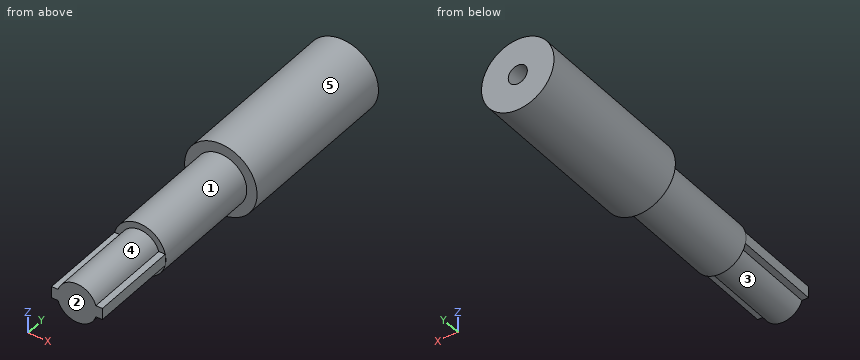
```python
from build123d import *

# Parameters (mm, degrees)
SKETCH1_R           = 3.1
SKETCH1_W           = 8
SKETCH1_H           = 1.8
BOSS_EXTRUDE1_DEPTH = 14
SKETCH2_R           = 4.075
BOSS_EXTRUDE2_DEPTH = 18
SKETCH3_R           = 5.7
BOSS_EXTRUDE3_DEPTH = 2
SKETCH4_R           = 5.7
BOSS_EXTRUDE4_DEPTH = 25
SKETCH5_R           = 1.5
CUT_EXTRUDE1_DEPTH  = 17


with BuildPart() as part:
    # Sketch1 → Boss-Extrude1 (new body)
    with BuildSketch(Plane(origin=(0, 0, 0), x_dir=(1, 0, 0), z_dir=(0, 1, 0))):
        Circle(SKETCH1_R)
        Rectangle(SKETCH1_W, SKETCH1_H)
    extrude(amount=BOSS_EXTRUDE1_DEPTH)

    # Sketch2 → Boss-Extrude2 (add)
    with BuildSketch(Plane(origin=(0, 14, 0), x_dir=(1, 0, 0), z_dir=(0, 1, 0))):
        with Locations(Location((0, 0, 0), (0, 0, 12.759485069))):
            Circle(SKETCH2_R)
    extrude(amount=BOSS_EXTRUDE2_DEPTH)

    # Sketch3 → Boss-Extrude3 (add)
    with BuildSketch(Plane(origin=(0, 32, 0), x_dir=(1, 0, 0), z_dir=(0, 1, 0))):
        with Locations(Location((0, 0, 0), (0, 0, 270))):
            Circle(SKETCH3_R)
    extrude(amount=BOSS_EXTRUDE3_DEPTH)

    # Sketch4 → Boss-Extrude4 (add)
    with BuildSketch(Plane(origin=(0, 34, 0), x_dir=(1, 0, 0), z_dir=(0, 1, 0))):
        with Locations(Location((0, 0, 0), (0, 0, 270))):
            Circle(SKETCH4_R)
    extrude(amount=BOSS_EXTRUDE4_DEPTH)

    # Sketch5 → Cut-Extrude1 (cut)
    with BuildSketch(Plane(origin=(0, 59, 0), x_dir=(1, 0, 0), z_dir=(0, 1, 0))):
        with Locations(Location((0, 0, 0), (0, 0, 270))):
            Circle(SKETCH5_R)
    extrude(amount=-CUT_EXTRUDE1_DEPTH, mode=Mode.SUBTRACT)


solid = part.part
```
The model under review builds one solid part; all positions refer to its coordinate system, in mm. Face numbers are marked on the shaded views. A direction names the side the tool comes from. Give positions to 0.01 mm unless a question says otherwise; leave off trailing zeros. Order: outer loops, then holes, each group sorted by start corner. A loop starts at its lowest first (then second) coordinate and runs counter-clockwise, first axis right, second up. Notation, with made-up numbers: (62, 86.25) - (101, 86.25) arc R12 ccw to (101, 95.25) - close; hole circle Ø5 at (-37.75, 75.25). An arc over 180 degrees is marked (long way). Use CSV: the item, a comma, the result in double quotes. Start each with the question number.
Q1. We need section D-D, the plane y = 33.5. Write out the cut boundary in (x, z), and give its area (3 significant figures).
Q2. Tool access review of the marked faces 4 and 5: name each direction out of +Z, -Z, +X, -X, +Y, -Y from which nothing blocks a thin tool from reaching the whole face with its end or side.
Q3. We need section C-C, the plane y = 45. Write out the cut boundary in (x, z).
Q4. The part is to be moulded in two halves that separate along Z. For the marked faces 1, 2 and 3, say which applies: +Z half, -Z half, draft (parallel to the pull), parting line (faces both ways), or undercut.
Q5. We need section B-B, the plane z = 0. Write out the cut boundary in (x, y) (3 decimals).
Q6. To check wall thickness, follow line 1 along X through (y, z) = (54.5, 0); line 2 along Y through (x, z) = (-3.75, 4.25); line 3 along Z through (x, y) = (0.5, 53.5). State the ranges of each line that lie inside material, in increasing order. Write a range as [from, to].
Q7. Clearance check with flat-ended pins moving along their axes: pin 1 Ø1.5 at (x, z) = (-0.5, -0.5) entering from +Y; pin 2 Ø2 at (x, y) = (-4, 16.5) entering from -Z; pin 3 Ø0.5 at (y, z) = (10, 0) entering from +X. State where each tip first meets the part, or that it passes through.
Q8. We need section A-A, the plane x = 0. Write out the cut boundary in (y, z) (3 decimals).
Outcome:
1,outline,"circle Ø11.4 at (0, 0)"
1,area,"102 mm^2"
2,face 4,"+Z, -Y"
2,face 5,"+Y, -Y"
3,outline,"circle Ø11.4 at (0, 0); hole circle Ø3 at (0, 0)"
4,face 1,"parting line"
4,face 2,"draft"
4,face 3,"-Z half"
5,outline,"(-5.7, 32) - (-4.075, 32) - (-4.075, 14) - (-4, 14) - (-4, 0) - (4, 0) - (4, 14) - (4.075, 14) - (4.075, 32) - (5.7, 32) - (5.7, 59) - (1.5, 59) - (1.5, 42) - (-1.5, 42) - (-1.5, 59) - (-5.7, 59) - close"
6,line 1,"x = [-5.7, -1.5], [1.5, 5.7]"
6,line 2,"y = [32, 59]"
6,line 3,"z = [-5.68, -1.41], [1.41, 5.68]"
7,pin 1,"stops at y = 42"
7,pin 2,"stops at z = -2.76"
7,pin 3,"stops at x = 4"
8,outline,"(0, -3.1) - (14, -3.1) - (14, -4.075) - (32, -4.075) - (32, -5.7) - (59, -5.7) - (59, -1.5) - (42, -1.5) - (42, 1.5) - (59, 1.5) - (59, 5.7) - (32, 5.7) - (32, 4.075) - (14, 4.075) - (14, 3.1) - (0, 3.1) - close"
